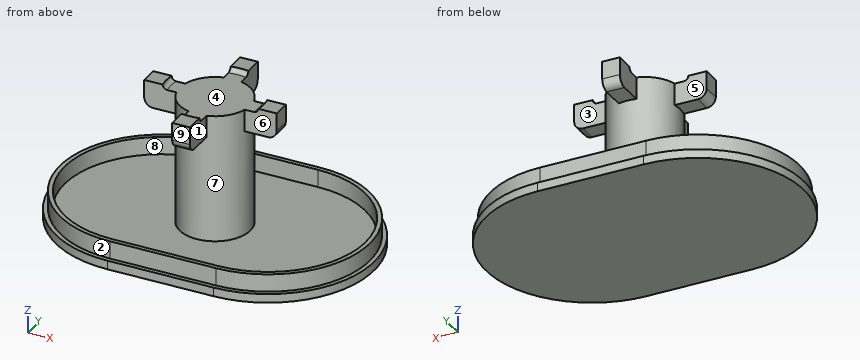
from build123d import *

# Parameters (mm, degrees)
F0_W      = 609.6
F0_H      = 25.4
F0_H_2    = 1117.6
F0_R      = 203.2
F1_DEPTH  = 50.8
F2_DEPTH  = 101.6
F3_DEPTH  = 762
F4_W      = 101.6
F4_H      = 152.4
F5_DEPTH  = 381
F6_W      = 101.6
F6_H      = 152.4
F7_DEPTH  = 381
F8_R      = 50.8
F9_R      = 279.4
F10_DEPTH = 25.4
F11_R     = 25.39999


# Not quite as in the source:
# - a fillet or chamfer is up to 0.001 mm smaller than in the source, because OpenCascade refuses the exact size


with BuildPart() as f1:
    # F0 (on Top) → F1 (new body)
    with BuildSketch(Plane.XY):
        with BuildLine():
            Line((-304.8, 584.2), (-304.8, 609.6))
            ThreePointArc((-304.8, 609.6), (-914.4, 0), (-304.8, -609.6))
            Line((-304.8, -609.6), (-304.8, -584.2))
            ThreePointArc((-304.8, -584.2), (-889, 0), (-304.8, 584.2))
        make_face()
        with BuildLine():
            Line((-304.8, 558.8), (-304.8, 584.2))
            ThreePointArc((-304.8, 584.2), (-889, 0), (-304.8, -584.2))
            Line((-304.8, -584.2), (-304.8, -558.8))
            ThreePointArc((-304.8, -558.8), (-863.6, 0), (-304.8, 558.8))
        make_face()
        with Locations((0, 596.9)):
            Rectangle(F0_W, F0_H)
        with BuildLine():
            ThreePointArc((304.8, -609.6), (914.4, 0), (304.8, 609.6))
            Line((304.8, 609.6), (304.8, 584.2))
            ThreePointArc((304.8, 584.2), (889, 0), (304.8, -584.2))
            Line((304.8, -584.2), (304.8, -609.6))
        make_face()
        with BuildLine():
            ThreePointArc((304.8, -584.2), (889, 0), (304.8, 584.2))
            Line((304.8, 584.2), (304.8, 558.8))
            ThreePointArc((304.8, 558.8), (863.6, 0), (304.8, -558.8))
            Line((304.8, -558.8), (304.8, -584.2))
        make_face()
        with Locations((0, -596.9)):
            Rectangle(F0_W, F0_H)
        with Locations((0, -571.5)):
            Rectangle(F0_W, F0_H)
        Rectangle(F0_W, F0_H_2)
        Circle(F0_R, mode=Mode.SUBTRACT)
        with BuildLine():
            ThreePointArc((304.8, -558.8), (863.6, 0), (304.8, 558.8))
            Line((304.8, 558.8), (304.8, -558.8))
        make_face()
        with BuildLine():
            Line((-304.8, -558.8), (-304.8, 558.8))
            ThreePointArc((-304.8, 558.8), (-863.6, 0), (-304.8, -558.8))
        make_face()
        with Locations((0, 571.5)):
            Rectangle(F0_W, F0_H)
        Circle(F0_R)
    extrude(amount=-F1_DEPTH)

    # F0 (on Top) → F2 (join)
    with BuildSketch(Plane.XY):
        with BuildLine():
            Line((-304.8, 558.8), (-304.8, 584.2))
            ThreePointArc((-304.8, 584.2), (-889, 0), (-304.8, -584.2))
            Line((-304.8, -584.2), (-304.8, -558.8))
            ThreePointArc((-304.8, -558.8), (-863.6, 0), (-304.8, 558.8))
        make_face()
        with Locations((0, -571.5)):
            Rectangle(F0_W, F0_H)
        with Locations((0, 571.5)):
            Rectangle(F0_W, F0_H)
        with BuildLine():
            ThreePointArc((304.8, -584.2), (889, 0), (304.8, 584.2))
            Line((304.8, 584.2), (304.8, 558.8))
            ThreePointArc((304.8, 558.8), (863.6, 0), (304.8, -558.8))
            Line((304.8, -558.8), (304.8, -584.2))
        make_face()
    extrude(amount=F2_DEPTH)

    # F0 (on Top) → F3 (join)
    with BuildSketch(Plane.XY):
        Circle(F0_R)
    extrude(amount=F3_DEPTH)

    # F4 (on Front) → F5 (join, symmetric)
    with BuildSketch(Plane.XZ):
        with Locations((0, 685.8)):
            Rectangle(F4_W, F4_H)
    extrude(amount=F5_DEPTH, both=True)

    # F6 (on Right) → F7 (join, symmetric)
    with BuildSketch(Plane.YZ):
        with Locations((0, 685.8)):
            Rectangle(F6_W, F6_H)
    extrude(amount=F7_DEPTH, both=True)

    # F8
    f8_edges = [f1.edges().sort_by_distance(p)[0] for p in [
        (0, -381, 609.6),
        (-381, 0, 609.6),
        (0, 381, 609.6),
        (381, 0, 609.6),
    ]]
    fillet(f8_edges, radius=F8_R)

    # F9 (on face) → F10 (cut)
    with BuildSketch(Plane.XY.offset(762)):
        Circle(F9_R)
    extrude(amount=-F10_DEPTH, mode=Mode.SUBTRACT)

    # F11 (radius 25.4 in the source; OpenCascade refuses exactly that, so slightly less here)
    f11_edges = [f1.edges().sort_by_distance(p)[0] for p in [
        (279.4, 0, 736.6),
        (-279.4, 0, 736.6),
        (0, 279.4, 736.6),
        (0, -279.4, 736.6),
    ]]
    fillet(f11_edges, radius=F11_R)


solid = f1.part
Could you check a few things on this model? Use its own coordinates, in mm. Face numbers are marked on the shaded views. A direction names the side the tool comes from. Round coordinates to 2 decimals unless told otherwise and drop trailing zeros. Order: outer loops, then holes, each group sorted by start corner. A loop starts at its lowest first (then second) coordinate and runs counter-clockwise, first axis right, second up.
Q1. Which directions (+Z, -Z, +X, -X, +Y, -Y) give clear straight access to the entire face, cutting with the end or side of a thin tool? Please do the marked faces 5, 6, 7, 8 and 9.
Geometry says:
face 5: +Z, -X, +Y
face 6: +Z, +X, -Y
face 7: none
face 8: +Z
face 9: +Z, +X, -X, -Y
Q2. Thinking about a two-plate mould opening in X: for the marked faces 1, 2, 3 and 4, which applies, released by +X, released by -X, zero draft, split by the parting line, or undercut?
Geometry says:
face 1: released by +X
face 2: released by -X
face 3: zero draft
face 4: undercut
Q3. Please list where these lines run through material, in increasing order: probe 1 along X at (y, z) = (59, 8.5); probe 2 along Y at (x, z) = (-13.5, 384); probe 3 along Z at (x, y) = (73.5, 171).
Geometry says:
probe 1: x = -886.01 to -860.48, -194.45 to 194.45, 860.48 to 886.01
probe 2: y = -202.75 to 202.75
probe 3: z = -50.8 to 736.6
Q4. Imagine slicing it at A-A, the plane z = 38. List the corners of the cut face in (x, y) for me.
Geometry says:
outline: (-304.8, -584.2) - (304.8, -584.2) arc R584.2 ccw to (304.8, 584.2) - (-304.8, 584.2) arc R584.2 ccw to start; circle Ø406.4 at (0, 0); hole (-304.8, -558.8) - (304.8, -558.8) arc R558.8 ccw to (304.8, 558.8) - (-304.8, 558.8) arc R558.8 ccw to start
Q5. I'm going to push flat-ended pins straight in: P1, Ø8, axis at x = 88, z = 314.5, coming from the -Y side (3 decimals); P2, Ø6, axis at x = 662.5, y = -425.5, coming from the +Z side; P3, Ø2, axis at y = 170, z = 347.5, coming from the -X side. Where does each tip first touch, or does it pass through?
Geometry says:
P1: stops at y = -185.025
P2: stops at z = 101.6
P3: stops at x = -112.82
Q6. Imagine slicing it at D-D, the plane z = 360.5. List the corners of the cut face in (x, y) for me, then the cut area to 3 significant figures.
Geometry says:
outline: circle Ø406.4 at (0, 0)
area: 130,000 mm2
